Geometry check sheet. Reference: the model listing, model coordinates, mm. Face numbers are marked on the shaded views. A direction names the side the tool comes from. Coordinates: 2 decimals unless noted, no trailing zeros. Write each loop counter-clockwise with the first axis right and the second up, starting at its lowest first coordinate (ties: lowest second). Pieces come first, ordered by that corner, then holes. Notation, with made-up numbers: M -23.75,-34 L -6.75,-34 A23 cw -6.75,-2 Z; hole C 55,33 d7. An arc over 180 degrees is marked long. Answer as a JSON object with one key per item and string values. Group by question number.
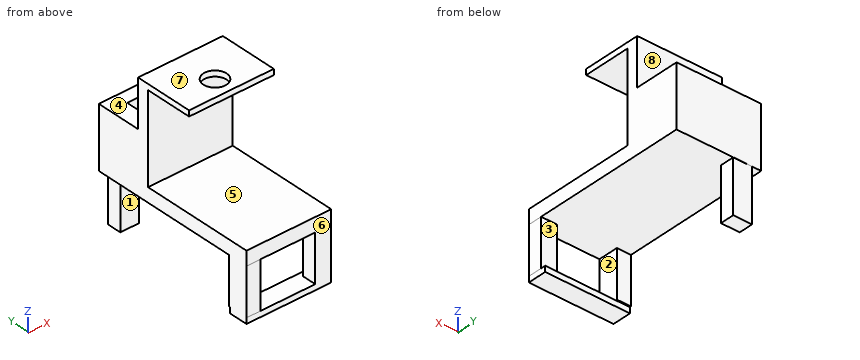
```python
from build123d import *

# Parameters (mm, degrees)
F0_W      = 45
F0_H      = 90
F1_DEPTH  = 7.5
F2_W      = 45
F2_H      = 30
F2_W_2    = 28.085665
F2_H_2    = 17
F3_DEPTH  = 25
F5_DEPTH  = 25
F6_W      = 45
F6_H      = 3
F7_DEPTH  = 25
F8_R      = 6.14005
F9_DEPTH  = 3
F10_W     = 8.500325
F10_H     = 7.5
F11_DEPTH = 25
F12_W     = 7.5
F12_H     = 10.662651
F13_DEPTH = 25
F14_W     = 10
F14_H     = 7.5
F15_DEPTH = 28
F16_W     = 45
F16_H     = 10
F17_DEPTH = 3


with BuildPart() as f1:
    # F0 (on Top) → F1 (new body)
    with BuildSketch(Plane.XY):
        Rectangle(F0_W, F0_H)
    extrude(amount=F1_DEPTH)

    # F2 (on face) → F3 (join)
    with BuildSketch(Plane.XY.offset(7.5)):
        with Locations((0, 30)):
            Rectangle(F2_W, F2_H)
        with Locations((0.5507, 29.56425)):
            Rectangle(F2_W_2, F2_H_2, mode=Mode.SUBTRACT)
    extrude(amount=F3_DEPTH)

    # F4 (on face) → F5 (join)
    with BuildSketch(Plane.XY.offset(32.5)):
        Polygon((-22.5, 15), (22.5, 15), (22.5, 21.06425), (14.593532, 21.06425), (-13.492133, 21.06425), (-22.5, 21.06425), align=None)
    extrude(amount=F5_DEPTH)

    # F6 (on face) → F7 (join)
    with BuildSketch(Plane.XZ.offset(-15)):
        with Locations((0, 56)):
            Rectangle(F6_W, F6_H)
    extrude(amount=F7_DEPTH)

    # F8 (on face) → F9 (cut, through all)
    with BuildSketch(Plane.XY.offset(57.5)):
        Circle(F8_R)
    extrude(amount=-F9_DEPTH, mode=Mode.SUBTRACT)

    # F10 (on face) → F11 (join)
    with BuildSketch(Plane(origin=(0, 0, 0), x_dir=(1, 0, 0), z_dir=(0, 0, -1))):
        with Locations((18.249837, 41.25)):
            Rectangle(F10_W, F10_H)
    extrude(amount=F11_DEPTH)

    # F12 (on face) → F13 (join)
    with BuildSketch(Plane(origin=(0, 0, 0), x_dir=(1, 0, 0), z_dir=(0, 0, -1))):
        with Locations((-18.75, 39.668674)):
            Rectangle(F12_W, F12_H)
    extrude(amount=F13_DEPTH)

    # F14 (on Top) → F15 (join)
    with BuildSketch(Plane.XY):
        with Locations((-12.690873, 41.181121)):
            Rectangle(F14_W, F14_H)
    extrude(amount=-F15_DEPTH)

    # F16 (on face) → F17 (join)
    with BuildSketch(Plane(origin=(0, 0, -25), x_dir=(1, 0, 0), z_dir=(0, 0, -1))):
        with Locations((0, 40)):
            Rectangle(F16_W, F16_H)
    extrude(amount=F17_DEPTH)


solid = f1.part
```
1) Set-up check for the marked faces 1, 2, 3, 4 and 5: record each of +Z, -Z, +X, -X, +Y, -Y from which the full face is reachable in a straight line by a thin tool's end or side.
2) Section check B-B (z = 15.5). Record the cut outline in (x, y), then the cut area to 3 significant figures.
3) Draft check along Y on the marked faces 6, 7 and 8. Enter one of: +Y half, -Y half, draft (parallel to the pull), parting line (faces both ways), or undercut.
4) Material ranges on probe 1 along Z at (x, y) = (20, -8); probe 2 along Y at (x, z) = (-7, 28.5); probe 3 along Y at (x, z) = (0, 56.1), recorded low to high. Write a range as [from, to].
5) Section check D-D (y = 0). Record the cut outline in (x, z), then the cut area to 3 significant figures.
6) Section check C-C (x = -9.5). Record the cut outline in (y, z).
7) Section check A-A (x = 0). Record the cut outline in (y, z).
8) Go/stop test with flat-tipped pins: pin 1 Ø8 at (x, y) = (-3.5, 1.5) entering from -Z; pin 2 Ø12 at (x, y) = (-9.5, 30) entering from +Z; pin 3 Ø12 at (x, z) = (13.5, 35.5) entering from -Y. Record where each tip stops, or that it passes through.
Entries:
{
 "1": {"face 1": "-Z, +X, -X", "face 2": "-Y", "face 3": "+X, +Y", "face 4": "+Z, +X, -X, +Y", "face 5": "+X, -X, -Y"},
 "2": {"outline": "M -22.5,15 L 22.5,15 L 22.5,45 L -22.5,45 Z; hole M -13.49,21.06 L 14.59,21.06 L 14.59,38.06 L -13.49,38.06 Z", "area": "873 mm^2"},
 "3": {"face 6": "-Y half", "face 7": "draft", "face 8": "undercut"},
 "4": {"probe 1": "[0, 7.5], [54.5, 57.5]", "probe 2": "[15, 21.06], [38.06, 45]", "probe 3": "[-10, -6.14], [6.14, 21.06]"},
 "5": {"outline": "M -22.5,0 L 22.5,0 L 22.5,7.5 L -22.5,7.5 Z; M -22.5,54.5 L -6.14,54.5 L -6.14,57.5 L -22.5,57.5 Z; M 6.14,54.5 L 22.5,54.5 L 22.5,57.5 L 6.14,57.5 Z", "area": "436 mm^2"},
 "6": {"outline": "M -45,-28 L -35,-28 L -35,-25 L -45,-25 Z; M -45,0 L 37.43,0 L 37.43,-28 L 44.93,-28 L 44.93,0 L 45,0 L 45,32.5 L 38.06,32.5 L 38.06,7.5 L 21.06,7.5 L 21.06,57.5 L -10,57.5 L -10,54.5 L 15,54.5 L 15,7.5 L -45,7.5 Z"},
 "7": {"outline": "M -45,-28 L -35,-28 L -35,-25 L -45,-25 Z; M -45,0 L 45,0 L 45,32.5 L 38.06,32.5 L 38.06,7.5 L 21.06,7.5 L 21.06,57.5 L 6.14,57.5 L 6.14,54.5 L 15,54.5 L 15,7.5 L -45,7.5 Z; M -10,54.5 L -6.14,54.5 L -6.14,57.5 L -10,57.5 Z"},
 "8": {"pin 1": "z = 0", "pin 2": "z = 32.5", "pin 3": "y = 15"}
}
